from build123d import *

# Parameters (mm, degrees)
F0_W        = 8.8490359485
F0_H        = 96.4175835252
F1_DEPTH    = 5.842
F2_T1_DEPTH = 121.8175835252


# Not quite as in the source:
# - a fillet or chamfer that OpenCascade refuses, or shapes differently, is made with other operations: its cross-section is extruded or revolved along the edge and cut away or added


with BuildPart() as f1:
    # F0 (on Front) → F1 (new body)
    with BuildSketch(Plane.XZ):
        with Locations((-62.4962914735, -2.8574988246)):
            Rectangle(F0_W, F0_H)
    extrude(amount=F1_DEPTH)

    # F2: fillet of radius 5.08 on 2 edges, made by hand

    # F2_s2 → F2_t1 (cut)
    with BuildSketch(Plane.XY.offset(-63.7662905872)):
        with BuildLine():
            ThreePointArc((-58.0717734993, -5.08), (-59.5596710508, -1.4878975516), (-63.1517734993, 0))
            Line((-63.1517734993, 0), (-58.0717734993, 0))
            Line((-58.0717734993, 0), (-58.0717734993, -5.08))
        make_face()
        with BuildLine():
            ThreePointArc((-66.9208094478, -5.08), (-65.4329118962, -1.4878975516), (-61.8408094478, 0))
            Line((-61.8408094478, 0), (-66.9208094478, 0))
            Line((-66.9208094478, 0), (-66.9208094478, -5.08))
        make_face()
    extrude(amount=F2_T1_DEPTH, mode=Mode.SUBTRACT)


solid = f1.part
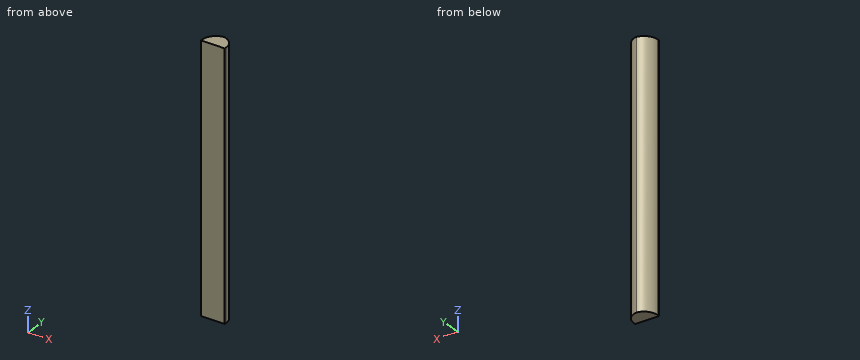
Can you work these out from the model? Positions are in its coordinate system, mm. Coordinates: 2 decimals unless noted, no trailing zeros. Order: outer loops, then holes, each group sorted by start corner. A loop starts at its lowest first (then second) coordinate and runs counter-clockwise, first axis right, second up. Notation, with made-up numbers: M 86,58 L 125,58 A9 cw 125,73 Z; hole C -31.5,26 d8. An arc over 180 degrees is marked long. Answer as CSV lines item,"result".
(1) Suppose I cut it at B-B on y = -2.9. Please give me the cut outline in (x, z), plus the area to 3 significant figures.
Geometry check:
outline,"M -66.43,-51.07 L -58.56,-51.07 L -58.56,45.35 L -66.43,45.35 Z"
area,"758 mm^2"
(2) Suppose I cut it at C-C on x = -59.5. Please give me the cut outline in (y, z), plus the area to 3 significant figures.
Geometry check:
outline,"M -5.84,-51.07 L -1.55,-51.07 L -1.55,45.35 L -5.84,45.35 Z"
area,"414 mm^2"
(3) I'm going to push flat-ended pins straight in: pin 1 (1 mm diameter, centred on y = -3.5, z = -40.5, fed in from +X); pin 2 (1 mm diameter, centred on y = -2.5, z = 6.5, fed in from +X). Where does each tip first touch, or does it pass through?
Geometry check:
pin 1,"x = -58.19"
pin 2,"x = -58.52"
(4) Please list where these lines run through material, in increasing order: L1, parallel to Y at x = -59.25, z = -0.5; L2, parallel to Y at x = -60.25, z = -32.5; L3, parallel to X at y = -1.4, z = 8.
Geometry check:
L1,"-5.84 to -1.83"
L2,"-5.84 to -0.91"
L3,"-65.34 to -59.65"
(5) Suppose I cut it at A-A on z = -39.5. Please give me the cut outline in (x, y).
Geometry check:
outline,"M -66.92,-5.84 L -58.07,-5.84 L -58.07,-5.08 A5.08 ccw -62.5,-0.04 A5.08 ccw -66.92,-5.08 Z"
